Geometry: see drawing. Coordinates: mm, zero at the bounding-box minimum. Give positions to 0.01 mm unless a question says otherwise; leave off trailing zeros. Write each loop counter-clockwise with the first axis right and the second up, starting at its lowest first coordinate (ties: lowest second). Pieces come first, ordered by that corner, then holes. Notation, with made-up numbers: (-38, -21) - (9, -21) arc R24 ccw to (9, -10) - close; hole circle Ø6 at (-18.75, 23.25). An arc over 180 degrees is marked (long way). Use a Markdown table: item, result. Add a question column.
1. Section query A-A, the plane z = 2.4. Return loops of the section in (x, y), plus the area to 3 significant figures.
2. Pin query (flat end, axial travel): pin 1 (5 mm diameter, centred on x = 34, y = 48.5, fed in from +Z); pin 2 (1.5 mm diameter, centred on y = 36, z = 1.5, fed in from +X); pin 3 (1.5 mm diameter, centred on x = 42.5, z = 3.5, fed in from -Y). Return the tip coordinate at first contact, or that it passes through.
3. Section query D-D, the plane y = 45. Return loops of the section in (x, z).
4. Material intervals for probe 1 along X at (y, z) = (8, 1.85); probe 2 along Y at (x, z) = (5, 3.5); probe 3 along Y at (x, z) = (51.5, 3.45), sorted ascending.
5. Section query B-B, the plane y = 8. Return loops of the section in (x, z), plus the area to 3 significant figures.
6. Section query C-C, the plane x = 5. Return loops of the section in (y, z), plus the area to 3 significant figures.
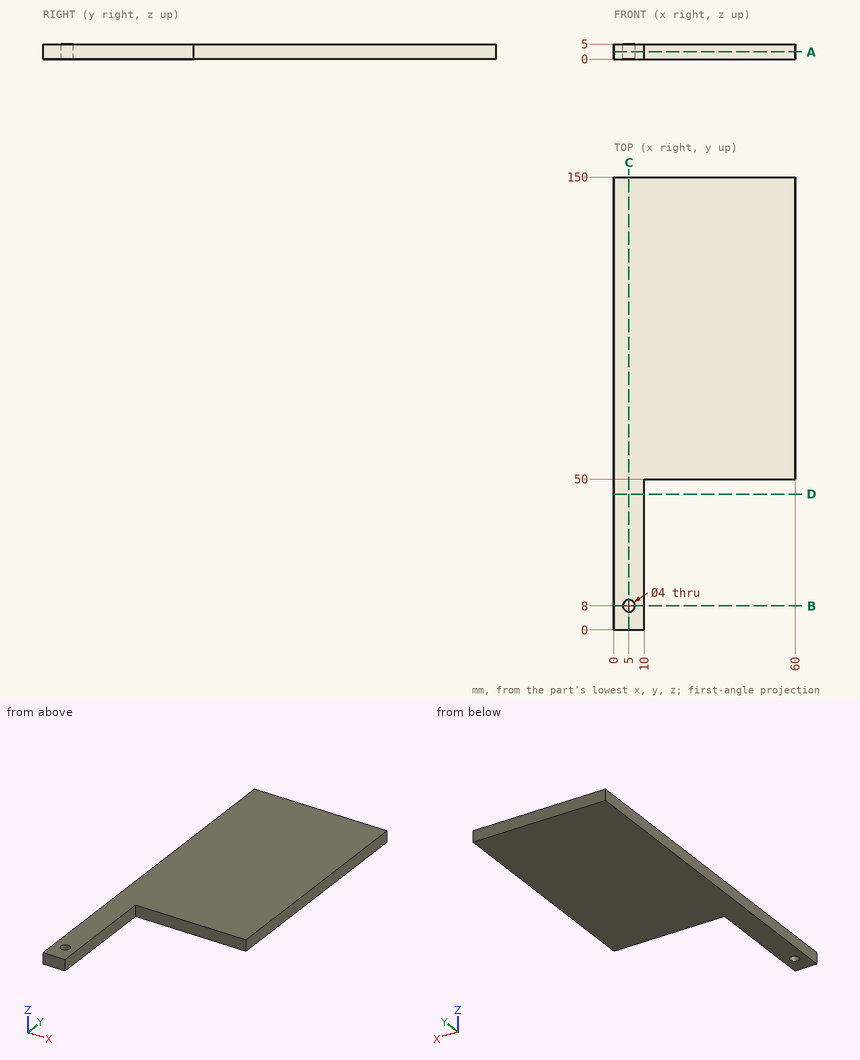
Result sheet:
| question | item | result |
|---|---|---|
| 1 | outline | (0, 0) - (10, 0) - (10, 50) - (60, 50) - (60, 150) - (0, 150) - close; hole circle Ø4 at (5, 8) |
| 1 | area | 6,490 mm² |
| 2 | pin 1 | stops at z = 5 |
| 2 | pin 2 | stops at x = 10 |
| 2 | pin 3 | stops at y = 50 |
| 3 | outline | (0, 0) - (10, 0) - (10, 5) - (0, 5) - close |
| 4 | probe 1 | x = 0 to 3, 7 to 10 |
| 4 | probe 2 | y = 0 to 6, 10 to 150 |
| 4 | probe 3 | y = 50 to 150 |
| 5 | outline | (0, 0) - (3, 0) - (3, 5) - (0, 5) - close; (7, 0) - (10, 0) - (10, 5) - (7, 5) - close |
| 5 | area | 30.0 mm² |
| 6 | outline | (0, 0) - (6, 0) - (6, 5) - (0, 5) - close; (10, 0) - (150, 0) - (150, 5) - (10, 5) - close |
| 6 | area | 730 mm² |
